Here's how the part is built. I have some questions about the finished solid (model axes, mm). Coordinates: 2 decimals unless noted, no trailing zeros. Loops run counter-clockwise (first coordinate to the right, second up) from the corner with the lowest first, then second, coordinate; pieces in that order, holes last. Notation, with made-up numbers: (-24.5, 50.5) -> (-7.5, 50.5) arc R31 ccw to (-7.5, 80.5) -> close; hole circle Ø9 at (9, -1.5). An arc over 180 degrees is marked (long way). Answer as a JSON object with one key per item and string values. Group by question number.
1) I want a section at A-A (y = 40). Write out the boundary of the cut face in (x, z).
2) I need wall thicknesses on probe 1 along Y at (x, z) = (40, 3.5); probe 2 along Y at (x, z) = (40, 0.5); probe 3 along X at (y, z) = (10, 4.5). Which ranges of each line are inside material? Lowest first, please. Write a range as [from, to].
3) I want a section at C-C (z = 1.35). Write out the boundary of the cut face in (x, y), then the cut area to 3 significant figures.
4) I want a section at B-B (x = 10). Write out the boundary of the cut face in (y, z), then the cut area to 3 significant figures.
5) I want a section at D-D (x = -50). Write out the boundary of the cut face in (y, z).
6) I'm going to push flat-ended pins straight in: pin 1 (5.5 mm diameter, centred on x = 40, y = 40, fed in from -Z); pin 2 (1.5 mm diameter, centred on y = 63.5, z = 0.5, fed in from +X); pin 3 (1 mm diameter, centred on x = 24.5, z = 1, fed in from +Y); pin 4 (2 mm diameter, centred on x = 18, z = 1.5, fed in from +Y). Where does each tip first touch, or does it pass through?
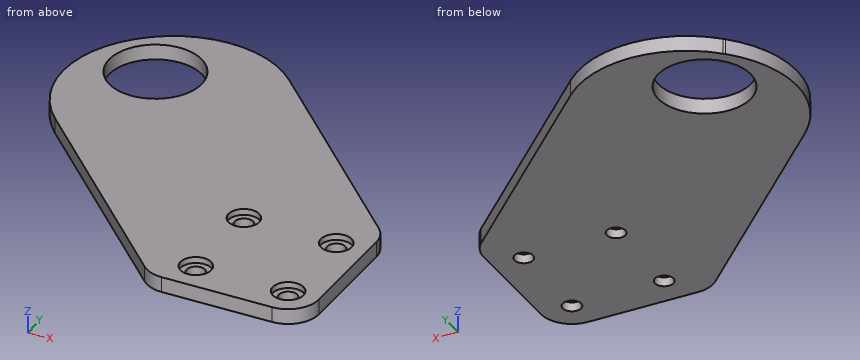
Autodesk Fusion 360 part; units mm, degrees
sketch "Sketch1" plane through (0, 0, 0) normal (0, 0, 1) x (1, 0, 0)
  line L0 (0, 0) -> (50, 0)
  line L1 (50, 0) -> (50, 50)
  line L2 (50, 50) -> (0, 50)
  line L3 (0, 50) -> (0, 0)
  dimension "d1" = 50
  dimension "d2" = 50
extrude "Extrude1" add sketch "Sketch1" along normal blind 5
sketch "Sketch2" plane through (0, 0, 0) normal (0, 0, 1) x (1, 0, 0)
  line L0 (0, 0) -> (50, 50)
  line L1 (50, 50) -> (-38.3883, 138.3883)
  line L2 (-38.3883, 138.3883) -> (-88.3883, 88.3883)
  line L3 (-88.3883, 88.3883) -> (0, 0)
  dimension "d5" = 125
extrude "Extrude2" add sketch "Sketch2" along normal blind 5
sketch "Sketch3" plane through (0, 0, 5) normal (0, 0, 1) x (-1, 0, 0)
  line L0 (0, 0) -> (-50, 0)
  line L1 (-50, 0) -> (-50, -50)
  line L2 (-50, -50) -> (38.3883, -138.3883)
  line L3 (38.3883, -138.3883) -> (88.3883, -88.3883)
  line L4 (88.3883, -88.3883) -> (0, 0)
  circle A0 centre (-10, -10) radius 5
  circle A1 centre (-40, -10) radius 5
  circle A2 centre (-40, -40) radius 5
  circle A3 centre (-10, -40) radius 5
  dimension "d8" = 10
  dimension "d9" = 10
  dimension "d10" = 10
  dimension "d11" = 10
extrude "Extrude3" cut sketch "Sketch3" against normal blind 2 contours A0 | A1 | A2 | A3
sketch "Sketch4" plane through (0, 0, 3) normal (0, 0, 1) x (-1, 0, 0)
  circle A0 centre (-10, -40) radius 5
  circle A1 centre (-10, -40) radius 3
  circle A2 centre (-40, -40) radius 3
  circle A3 centre (-10, -10) radius 3
  circle A4 centre (-40, -10) radius 3
  dimension "d14" = 6
  dimension "d15" = 6
  dimension "d16" = 6
  dimension "d17" = 6
extrude "Extrude4" cut sketch "Sketch4" against normal blind 5 contours A1 | A2 | A3 | A4
sketch "Sketch5" plane through (0, 0, 5) normal (0, 0, 1) x (-1, 0, 0)
  circle A0 centre (-40, -40) radius 5
  circle A1 centre (-40, -10) radius 5
  circle A2 centre (-10, -40) radius 5
  circle A3 centre (-10, -10) radius 5
  line L0 (0, 0) -> (-50, 0)
  line L1 (-50, 0) -> (-50, -50)
  line L2 (-50, -50) -> (38.3883, -138.3883)
  line L3 (38.3883, -138.3883) -> (88.3883, -88.3883)
  line L4 (88.3883, -88.3883) -> (0, 0)
  circle A4 centre (50, -100) radius 15
  dimension "d20" = 30
extrude "Extrude5" cut sketch "Sketch5" against normal blind 5 contours A4
fillet "Fillet1" radius 35 2 edges at (-88.3883, 88.3883, 2.5) (-38.3883, 138.3883, 2.5)
fillet "Fillet2" radius 10 3 edges at (0, 0, 2.5) (50, 0, 2.5) (50, 50, 2.5)
Determined:
{
 "1": {"outline": "(-40, 0) -> (7, 0) -> (7, 3) -> (5, 3) -> (5, 5) -> (-40, 5) -> close; (13, 0) -> (37, 0) -> (37, 3) -> (35, 3) -> (35, 5) -> (15, 5) -> (15, 3) -> (13, 3) -> close; (43, 0) -> (50, 0) -> (50, 5) -> (45, 5) -> (45, 3) -> (43, 3) -> close"},
 "2": {"probe 1": "[0, 5], [15, 35], [45, 60]", "probe 2": "[0, 7], [13, 37], [43, 60]", "probe 3": "[-10, 5], [15, 35], [45, 50]"},
 "3": {"outline": "(-63.64, 63.64) -> (-2.93, 2.93) arc R10 ccw to (4.14, 0) -> (40, 0) arc R10 ccw to (50, 10) -> (50, 45.86) arc R10 ccw to (47.07, 52.93) -> (-13.64, 113.64) arc R35 ccw to (-63.14, 113.64) -> (-63.64, 113.14) arc R35 ccw to start; hole circle Ø30 at (-50, 100); hole circle Ø6 at (10, 10); hole circle Ø6 at (10, 40); hole circle Ø6 at (40, 10); hole circle Ø6 at (40, 40)", "area": "8,720 mm^2"},
 "4": {"outline": "(0, 0) -> (7, 0) -> (7, 3) -> (5, 3) -> (5, 5) -> (0, 5) -> close; (13, 0) -> (37, 0) -> (37, 3) -> (35, 3) -> (35, 5) -> (15, 5) -> (15, 3) -> (13, 3) -> close; (43, 0) -> (90, 0) -> (90, 5) -> (45, 5) -> (45, 3) -> (43, 3) -> close", "area": "374 mm^2"},
 "5": {"outline": "(50, 0) -> (85, 0) -> (85, 5) -> (50, 5) -> close; (115, 0) -> (121.91, 0) -> (121.91, 5) -> (115, 5) -> close"},
 "6": {"pin 1": "through", "pin 2": "x = 37.25", "pin 3": "y = 76", "pin 4": "y = 83"}
}
